Autodesk Inventor part; units mm, degrees
ref_plane "作業平面2" through (0, 0, 0) normal (1, 0, 0) x (0, 0, -1)
ref_plane "YZ Plane" through (0, 0, 0) normal (1, 0, 0) x (0, 1, 0)
ref_plane "XZ Plane" through (0, 0, 0) normal (0, 1, 0) x (-1, 0, 0)
sketch "スケッチ1" plane through (0, 0, 0) normal (0, 1, 0) x (-1, 0, 0)
  arc A0 (0.9, 0) -> (-0.9, 0) centre (0, 0) ccw
  arc A1 (-0.9, -4) -> (0.9, -4) centre (0, -4) ccw
  line L0 (0, 0) -> (0, -4) construction
  line L1 (-0.9, -4) -> (-0.9, 0)
  line L2 (0.9, -4) -> (0.9, 0)
  arc A2 (-2.5, -4) -> (2.5, -4) centre (0, -4) ccw
  line L3 (-2.5, -4) -> (-2.5, 0)
  arc A3 (2.5, 0) -> (-2.5, 0) centre (0, 0) ccw
  line L4 (2.5, 0) -> (2.5, -4)
  line L5 (8.4, -3.5) -> (2.5, -3.5)
  line L6 (2, 1.5) -> (8.4, 1.5)
  line L7 (8.4, 1.5) -> (8.4, -3.5)
  line L8 (8.4, -3.5) -> (3.4, -3.5)
  line L9 (3.4, -3.5) -> (3.4, 1.5)
  line L10 (3.4, 1.5) -> (8.4, 1.5)
  line L11 (8.4, 1.5) -> (8.4, -3.5)
  point P0 (2.5, -2.5)
  point P1 (-2.5, -2.5)
  point P2 (1.2097, 2.1879)
  point P3 (5.9, -3.5)
  point P4 (5.9, -3.5)
  point P5 (3.4, -3.5)
  point P6 (0, 2.5)
  dimension "d0" = 1.8
  dimension "d1" = 4
  dimension "d2" = 1.6
  dimension "d6" = 5
  dimension "d27" = 5.9
  dimension "d28" = 5
  dimension "d46" = 1
extrude "押し出し1" add sketch "スケッチ1" along normal blind 2
extrude "押し出し4" add sketch "スケッチ1" against normal blind 8 contours L9 L6 L7 L5
sketch "スケッチ5" plane through (-8.4, 2, -3.5) normal (-1, 0, 0) x (0, 0, 1)
  line L0 (5, -10) -> (0, -10)
  point P0 (3.5, -2)
  point P1 (2.5, -7.8)
  point P2 (2.5, -10)
  dimension "d31" = 2.2
hole "穴2" at (-8.4, -5.8, -1) direction (1, 0, 0) diameter 2.2 end through all
fillet "フィレット2" radius 1 1 edges at (-3.4, 0, -1)
ref_plane "作業平面2" through (0, 0, 0) normal (1, 0, 0) x (0, 0, -1)
chamfer "面取り1" distance 1 angle 45 2 edges at (-8.4, -8, -1) (-3.4, -8, -1)
sketch "スケッチ6" plane through (0, -8, 0) normal (0, -1, 0) x (1, 0, 0)
  line L0 (-4.4, 1.5) -> (-4.4, -3.5)
  line L1 (-7.4, -3.5) -> (-7.4, 1.5)
  line L2 (-7.4, -0.25) -> (-4.4, -0.25)
  line L3 (-4.4, -0.25) -> (-4.4, -1.75)
  line L4 (-4.4, -1.75) -> (-7.4, -1.75)
  line L5 (-7.4, -1.75) -> (-7.4, -0.25)
  point P0 (0, 0)
  point P1 (-7.4, -1)
  point P2 (-7.4, -1.75)
  point P3 (-4.4, -0.25)
  dimension "d43" = 1.5
extrude "押し出し5" add sketch "スケッチ6" along normal blind 1
properties part number "om_Drop" material "ABS プラスチック"
Design review of the part built by this model. Coordinates are the model's own, in mm. A direction names the side the tool comes from. Give positions to 0.01 mm unless a question says otherwise; leave off trailing zeros. Loops run counter-clockwise (first coordinate to the right, second up) from the corner with the lowest first, then second, coordinate; pieces in that order, holes last. Notation, with made-up numbers: M 5.25,22 L 11.25,22 A18 ccw 11.25,48 Z; hole C -6.75,10.25 d9. An arc over 180 degrees is marked long. Return JSON: item names as keys, results as strings. Group by question number.
Item 1: Insertion check: pin 1 Ø1 at (x, z) = (-1.5, 0.5) entering from -Y; pin 2 Ø0.5 at (y, z) = (-8.5, -0.5) entering from +X; pin 3 Ø6 at (x, y) = (-5.5, -6) entering from -Z. Each pin has a flat end and moves straight along its axis. Give the tip position at first contact, or say it passes through.
Item 2: We need section D-D (y = -5.8). Give the boundary of the cut face in (x, z), and give its area (3 significant figures).
Item 3: Mouldability with a two-part tool opening along X and no side actions: class faces 1 (the flat face through (-7.9, -7.5, -1)), 2 (the flat face through (-5.9, -8.5, -0.25)), 3 (the flat face through (0.9, 1, -2)) as released by +X, released by -X, zero draft, split by the parting line, or undercut.
Item 4: Tool access review of faces 4 (the flat face through (-5.9, -8.5, -1.75)), 5 (the flat face through (-6, -3, 1.5)), 6 (the flat face through (1.2, 0, -1.9)), 7 (the flat face through (-5, -3, -3.5)), 8 (the flat face through (-6, -8, 1)): name each direction out of +Z, -Z, +X, -X, +Y, -Y from which nothing blocks a thin tool from reaching the whole face with its end or side.
Item 5: We need section B-B (y = 1). Give the boundary of the cut face in (x, z).
Item 6: We need section A-A (z = -1). Give the boundary of the cut face in (x, y), and give its area (3 significant figures).
Item 7: For probe 1 along X at (y, z) = (1.5, -3); probe 2 along Z at (x, y) = (-5.2, -5.8); probe 3 along Y at (x, z) = (-5, -1), list the stretches that pass through material, from the lowest coordinate up.
Item 8: We need section C-C (x = 0). Give the boundary of the cut face in (y, z).
Output:
{
 "1": {"pin 1": "stops at y = 0", "pin 2": "stops at x = -4.4", "pin 3": "stops at z = -3.5"},
 "2": {"outline": "M -8.4,-3.5 L -3.4,-3.5 L -3.4,-2.1 L -8.4,-2.1 Z; M -8.4,0.1 L -3.4,0.1 L -3.4,1.5 L -8.4,1.5 Z", "area": "14.0 mm^2"},
 "3": {"face 1": "released by -X", "face 2": "zero draft", "face 3": "undercut"},
 "4": {"face 4": "-Z, +X, -X, -Y", "face 5": "+Z, -X, +Y, -Y", "face 6": "+Z, -Z, +X, -Y", "face 7": "-Z, -X, +Y, -Y", "face 8": "+Z, +X, -X, -Y"},
 "5": {"outline": "M -8.4,-3.5 L -2.5,-3.5 L -2.5,-4 A2.5 ccw 2.5,-4 L 2.5,0 A2.5 ccw -2,1.5 L -8.4,1.5 Z; hole M -0.9,-4 A0.9 ccw 0.9,-4 L 0.9,0 A0.9 ccw -0.9,0 Z"},
 "6": {"outline": "M -8.4,-7 L -7.4,-8 L -7.4,-9 L -4.4,-9 L -4.4,-8 L -3.4,-7 L -3.4,-6.9 L -8.4,-6.9 Z; M -8.4,-4.7 L -3.4,-4.7 L -3.4,-1 A1 cw -2.4,0 L -0.9,0 L -0.9,2 L -8.4,2 Z; M 0.9,0 L 2.5,0 L 2.5,2 L 0.9,2 Z", "area": "49.4 mm^2"},
 "7": {"probe 1": "x = -8.4 to -0.9, 0.9 to 2.5", "probe 2": "z = -3.5 to -2.1, 0.1 to 1.5", "probe 3": "y = -9 to -6.9, -4.7 to 2"},
 "8": {"outline": "M 0,-6.5 L 2,-6.5 L 2,-4.9 L 0,-4.9 Z; M 0,0.9 L 2,0.9 L 2,2.5 L 0,2.5 Z"}
}
